Autodesk Inventor part; units mm, degrees
ref_plane "Flange Pattern Plane" through (31.75, 7.5406, -4.5466) normal (0, 1, 0) x (1, 0, 0)
ref_plane "YZ Plane" through (0, 0, 0) normal (1, 0, 0) x (0, 1, 0)
ref_plane "XZ Plane" through (0, 0, 0) normal (0, 1, 0) x (-1, 0, 0)
sketch "Sketch1" plane through (0, 0, 0) normal (0, 1, 0) x (-1, 0, 0)
  line L0 (-31.75, 0) -> (31.75, 0)
  line L1 (31.75, 0) -> (31.75, -12.7)
  line L2 (31.75, -12.7) -> (-31.75, -12.7)
  line L3 (-31.75, -12.7) -> (-31.75, 0)
  line L4 (31.75, 0) -> (-31.75, -12.7) construction
  point P0 (0, 0)
  point P1 (0, 0)
  dimension "d0" = 63.5
  dimension "d1" = 12.7
extrude "Plate1" add sketch "Sketch1" along normal blind 1.1906
sketch "Sketch2" plane through (30.5594, 0, -12.7) normal (1, 0, 0) x (0, 1, 0)
  line L0 (0, 12.7) -> (0, 0)
  line L1 (0, 0) -> (13.8906, 0)
  line L2 (13.8906, 0) -> (13.8906, 12.7)
  line L3 (13.8906, 12.7) -> (0, 12.7)
edge flange "Flanges" height 12.7 angle 90 thickness 1.1906 bend radius 0.7937 thickness toward (1, 0, 0) relief tear relief width 1.1906 relief depth 0.5953 corner gap 1.1906 corner form 0 edges at (31.75, 1.1906, -6.35) (-31.75, 1.1906, -6.35) wall of the first edge with corners at (30.5594, 0, 0) (30.5594, 0, -12.7) (30.5594, 13.8906, -12.7) (30.5594, 13.8906, 0)
bend "Bend1"
corner "Corner1"
sketch "Sketch3" plane through (31.75, 1.9844, -12.7) normal (1, 0, 0) x (0, 0, -1)
  line L0 (-8.1534, 7.8677) -> (-4.5466, 7.8677)
  line L1 (-4.0386, 7.3597) -> (-4.0386, 3.7529)
  line L2 (-4.5466, 3.2449) -> (-8.1534, 3.2449)
  line L3 (-8.6614, 3.7529) -> (-8.6614, 7.3597)
  arc A0 (-8.1534, 7.8677) -> (-8.6614, 7.3597) centre (-8.1534, 7.3597) ccw
  arc A1 (-4.0386, 7.3597) -> (-4.5466, 7.8677) centre (-4.5466, 7.3597) ccw
  arc A2 (-4.5466, 3.2449) -> (-4.0386, 3.7529) centre (-4.5466, 3.7529) ccw
  arc A3 (-8.6614, 3.7529) -> (-8.1534, 3.2449) centre (-8.1534, 3.7529) ccw
  line L4 (-12.7, 0) -> (-12.7, 11.9063) construction
  line L5 (-12.7, 11.9063) -> (0, 11.9063) construction
  line L6 (-8.1534, 7.3597) -> (-4.5466, 3.7529) construction
  point P0 (-12.7, -1.9844)
  point P1 (-4.0386, 3.2449)
  point P2 (-8.6614, 3.2449)
  point P3 (-6.35, 5.5563)
  dimension "d16" = 4.6228
  dimension "d17" = 0.508
  dimension "d20" = 6.35
  dimension "d21" = 6.35
extrude "Flange Stamp" cut sketch "Sketch3" against normal blind 1.1906
sketch "Sketch7" plane through (31.75, 1.9844, 0) normal (1, 0, 0) x (0, 0, -1)
  arc A0 (4.5466, 7.8677) -> (4.0386, 7.3597) centre (4.5466, 7.3597) ccw construction
  arc A1 (8.1534, 3.2449) -> (8.6614, 3.7529) centre (8.1534, 3.7529) ccw construction
  circle A2 centre (6.35, 5.5563) radius 2.1844
  line L0 (4.5466, 7.3597) -> (8.1534, 3.7529) construction
  point P0 (0, -1.9844)
  dimension "d46" = 4.3688
surface extrude "Flange Circle" sketch "Sketch7" against normal up to surface (1.1906 mm away) shown yes curves A2
ref_plane "Flange Pattern Plane" through (31.75, 7.5406, -4.5466) normal (0, 1, 0) x (1, 0, 0)
feature "Flange Pattern" [suppressed]
sketch "Sketch8" plane through (0, 0, 0) normal (0, -1, 0) x (1, 0, 0)
  line L0 (29.7656, 0) -> (-29.7656, 0) construction
  line L1 (27.2034, -4.0386) -> (23.5966, -4.0386)
  line L2 (23.0886, -4.5466) -> (23.0886, -8.1534)
  line L3 (23.5966, -8.6614) -> (27.2034, -8.6614)
  line L4 (27.7114, -8.1534) -> (27.7114, -4.5466)
  arc A0 (27.7114, -4.5466) -> (27.2034, -4.0386) centre (27.2034, -4.5466) ccw
  arc A1 (27.2034, -8.6614) -> (27.7114, -8.1534) centre (27.2034, -8.1534) ccw
  arc A2 (23.0886, -8.1534) -> (23.5966, -8.6614) centre (23.5966, -8.1534) ccw
  arc A3 (23.5966, -4.0386) -> (23.0886, -4.5466) centre (23.5966, -4.5466) ccw
  line L5 (27.2034, -4.5466) -> (23.5966, -8.1534) construction
  line L6 (31.75, 0) -> (31.75, -12.7) construction
  point P0 (0, 0)
  point P1 (23.0886, -8.6614)
  point P2 (27.7114, -8.6614)
  point P3 (25.4, -6.35)
  dimension "d49" = 4.6228
  dimension "d50" = 0.508
  dimension "d51" = 6.35
  dimension "d52" = 6.35
extrude "Body Stamp" cut sketch "Sketch8" against normal blind 1.1906
sketch "Sketch9" plane through (0, 0, 0) normal (0, -1, 0) x (1, 0, 0)
  arc A0 (27.7114, -4.5466) -> (27.2034, -4.0386) centre (27.2034, -4.5466) ccw construction
  arc A1 (23.0886, -8.1534) -> (23.5966, -8.6614) centre (23.5966, -8.1534) ccw construction
  line L0 (27.2034, -4.5466) -> (23.5966, -8.1534) construction
  circle A2 centre (25.4, -6.35) radius 2.1844
  point P0 (0, 0)
  dimension "d55" = 4.3688
surface extrude "Body Circle" sketch "Sketch9" against normal up to surface (1.1906 mm away) shown yes curves A2
feature "Body Pattern" [suppressed]
sketch "Arc Length" plane through (30.5594, 1.9844, 0) normal (0, 0, 1) x (1, 0, 0)
  line L0 (0, 0) -> (1.1906, 0) construction
  arc A0 (-0.7938, -0.7938) -> (0, 0) centre (-0.7938, 0) ccw construction
  line L1 (-0.7938, -1.9844) -> (-0.7938, -0.7938) construction
  arc A1 (-0.7938, -1.9844) -> (1.1906, 0) centre (-0.7938, 0) ccw construction
  point P0 (-30.5594, -1.9844)
  dimension "d85" = 3.117
  dimension "d92" = 1.2468
sketch "Sketch13" plane through (31.75, 13.8906, 0) normal (1, 0, 0) x (0, 0, -1)
  line L0 (0, 0) -> (12.7, 0) construction
  line L1 (62.4078, 0) -> (63.4238, -1.016)
  line L2 (63.4238, -1.016) -> (64.4398, 0)
  line L3 (62.4078, 0) -> (64.4398, 0)
  line L4 (12.7, -11.9063) -> (0, -11.9063) construction
  line L5 (63.4238, -10.8903) -> (61.3168, -12.9972)
  line L6 (61.3168, -12.9972) -> (63.4238, -15.1042)
  line L7 (63.4238, -15.1042) -> (65.5308, -12.9972)
  line L8 (65.5308, -12.9972) -> (63.4238, -10.8903)
  line L9 (63.4238, -10.8903) -> (63.4238, -15.1042) construction
  line L10 (63.4238, -1.016) -> (63.4238, -10.8903) construction
  line L11 (0, -11.9063) -> (12.7, -11.9063) construction
  point P0 (0, -13.8906)
  dimension "d86" = 4.2139
  dimension "d88" = 1.016
  dimension "d91" = 1.016
  dimension "d102" = 63.4238
feature "Notch" [suppressed]
mirror "Notch Mirror" [suppressed]
pattern_linear "Notch Pattern" [suppressed]
chamfer "End Chamfer" distance 1.016 angle 45 4 edges at (-31.1547, 13.8906, -12.7) (31.1547, 13.8906, -12.7) (-31.1547, 13.8906, 0) (31.1547, 13.8906, 0)
sketch "Sketch14" plane through (-31.75, 1.9844, 431.8) normal (1, 0, 0) x (0, 0, -1)
  line L0 (431.8, 11.9063) -> (444.5, 11.9063) construction
  line L1 (431.8, 0) -> (431.8, 11.9063) construction
  line L2 (431.8, -1.9844) -> (444.5, -1.9844) construction
  line L3 (431.8, 11.9063) -> (444.5, 11.9063)
  line L4 (444.5, 11.9063) -> (444.5, -1.9844)
  line L5 (444.5, -1.9844) -> (431.8, -1.9844)
  line L6 (431.8, -1.9844) -> (431.8, 11.9063)
  point P0 (382.0521, -1.9844)
extrude "Half Cut" cut sketch "Sketch14" along normal blind 50.8
sketch "Flange Pattern Sketch" plane through (31.75, 7.5406, -4.5466) normal (0, 1, 0) x (1, 0, 0)
  line L0 (0, 3.6068) -> (0, 0) construction
  line L1 (-76.2822, -4.5466) -> (13.1932, -4.5466) construction
  line L2 (0, 0) -> (-1.1906, 0) construction
  point P0 (-31.75, -4.5466)
  point P1 (0, 1.8034)
  point P2 (0, 14.5034)
  point P3 (0, 27.2034)
  point P4 (0, 39.9034)
  point P5 (0, 52.6034)
  point P6 (0, 65.3034)
  point P7 (0, 78.0034)
  point P8 (0, 90.7034)
  point P9 (0, 103.4034)
  point P10 (0, 116.1034)
  point P11 (0, 128.8034)
  point P12 (0, 141.5034)
  point P13 (0, 154.2034)
  point P14 (0, 166.9034)
  point P15 (0, 179.6034)
  point P16 (0, 192.3034)
  point P17 (0, 205.0034)
  point P18 (0, 217.7034)
  point P19 (0, 230.4034)
  point P20 (0, 243.1034)
  point P21 (0, 255.8034)
  point P22 (0, 268.5034)
  point P23 (0, 281.2034)
  point P24 (0, 293.9034)
  point P25 (0, 306.6034)
  point P26 (0, 319.3034)
  point P27 (0, 332.0034)
  point P28 (0, 344.7034)
  point P29 (0, 357.4034)
  point P30 (0, 370.1034)
  point P31 (0, 382.8034)
  point P32 (0, 395.5034)
  point P33 (0, 408.2034)
  point P34 (0, 420.9034)
  point P35 (0, 433.6034)
  dimension "d131" = 12.7
  dimension "d134" = 12.7
sketch "Body Pattern Sketch" plane through (0, 0, 0) normal (0, -1, 0) x (1, 0, 0)
  line L0 (29.7656, 0) -> (-29.7656, 0) construction
  line L1 (31.75, 0) -> (31.75, -12.7) construction
  circle A0 centre (25.4, -6.35) radius 2.1844 construction
  point P0 (0, 0)
  point P1 (25.4, -19.05)
  point P2 (25.4, -31.75)
  point P3 (25.4, -44.45)
  point P4 (25.4, -57.15)
  point P5 (25.4, -69.85)
  point P6 (25.4, -82.55)
  point P7 (25.4, -95.25)
  point P8 (25.4, -107.95)
  point P9 (25.4, -120.65)
  point P10 (25.4, -133.35)
  point P11 (25.4, -146.05)
  point P12 (25.4, -158.75)
  point P13 (25.4, -171.45)
  point P14 (25.4, -184.15)
  point P15 (25.4, -196.85)
  point P16 (25.4, -209.55)
  point P17 (25.4, -222.25)
  point P18 (25.4, -234.95)
  point P19 (25.4, -247.65)
  point P20 (25.4, -260.35)
  point P21 (25.4, -273.05)
  point P22 (25.4, -285.75)
  point P23 (25.4, -298.45)
  point P24 (25.4, -311.15)
  point P25 (25.4, -323.85)
  point P26 (25.4, -336.55)
  point P27 (25.4, -349.25)
  point P28 (25.4, -361.95)
  point P29 (25.4, -374.65)
  point P30 (25.4, -387.35)
  point P31 (25.4, -400.05)
  point P32 (25.4, -412.75)
  point P33 (25.4, -425.45)
  point P34 (25.4, -438.15)
  dimension "d62" = 12.7
  dimension "d65" = 12.7
  dimension "d139" = 12.7
equation "\"d1\" = 1.27 * Length"
equation "\"d18\" = Thickness"
equation "\"d53\" = Thickness"
equation "\"d89\" = Thickness"
equation "\"d2\" = Thickness"
equation "\"d3\" = BendReliefWidth"
equation "\"d4\" = BendReliefDepth"
equation "\"d5\" = MinimumRemnant"
equation "\"d6\" = TransitionRadius"
equation "\"d10\" = CornerReliefSize"
equation "\"d11\" = GapSize"
equation "\"d12\" = JacobiRadiusSize"
equation "\"BendRadius\" = Thickness"
equation "\"BendReliefWidth\" = Thickness"
equation "\"BendReliefDepth\" = 0.5 * Thickness"
equation "\"CornerReliefSize\" = 4 * Thickness"
equation "\"MinimumRemnant\" = 2 * Thickness"
equation "\"TransitionRadius\" = BendRadius"
equation "\"JacobiRadiusSize\" = BendRadius"
equation "\"GapSize\" = Thickness"
properties part number "Alu C 1x3x1x35"
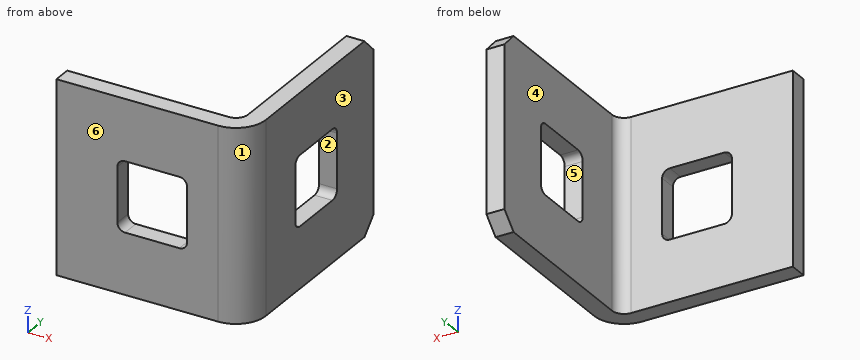
Design review of the part built by this model. Coordinates are the model's own, in mm. Face numbers are marked on the shaded views. A direction names the side the tool comes from. Give positions to 0.01 mm unless a question says otherwise; leave off trailing zeros. Write each loop counter-clockwise with the first axis right and the second up, starting at its lowest first coordinate (ties: lowest second). Pieces come first, ordered by that corner, then holes. Notation, with made-up numbers: M 73,37.5 L 103,37.5 A19 ccw 103,66.5 Z; hole C -4.75,46 d2. An arc over 180 degrees is marked long. Return JSON: item names as keys, results as strings. Group by question number.
Item 1: Take a section at C-C (y = 6). Give the boundary of the cut face in (x, z).
Item 2: Wall thickness on line 1 along Y through (x, z) = (26.25, -4); line 2 along X through (y, z) = (9, -1.25); line 3 along Y through (x, z) = (30.25, -3.5): over which ranges is each line inside the solid? List them lowest first.
Item 3: Take a section at D-D (z = -10.5). Give the boundary of the cut face in (x, y), plus the area to 3 significant figures.
Item 4: Tool access review of the marked faces 4, 5 and 6: name each direction out of +Z, -Z, +X, -X, +Y, -Y from which nothing blocks a thin tool from reaching the whole face with its end or side.
Item 5: Take a section at B-B (z = -6.5). Give the boundary of the cut face in (x, y), plus the area to 3 significant figures.
Item 6: Clearance check with flat-ended pins moving along their axes: pin 1 Ø1 at (x, y) = (26, 3) entering from +Z; pin 2 Ø3 at (x, y) = (30.5, 4.5) entering from -Z; pin 3 Ø1.5 at (y, z) = (3.5, -9) entering from -X; pin 4 Ø5 at (x, z) = (25.5, -2) entering from +Y. State where each tip first meets the part, or that it passes through.
Item 7: Take a section at A-A (x = 24). Give the boundary of the cut face in (y, z), plus the area to 3 significant figures.
Item 8: The part is to be moulded in two halves that separate along Y. For the marked faces 1, 2 and 3, say which applies: pulls with the +Y half, pulls with the -Y half, needs draft (parallel to the pull), parting line crosses it, or undercut.
Return value:
{
 "1": {"outline": "M 30.56,-12.7 L 31.75,-12.7 L 31.75,-8.66 L 30.56,-8.66 Z; M 30.56,-4.04 L 31.75,-4.04 L 31.75,0 L 30.56,0 Z"},
 "2": {"line 1": "y = 0 to 1.19", "line 2": "x = 30.56 to 31.75", "line 3": "y = 0.06 to 1.36"},
 "3": {"outline": "M 19.05,0 L 29.77,0 A1.98 ccw 31.75,1.98 L 31.75,13.89 L 30.56,13.89 L 30.56,1.98 A0.79 cw 29.77,1.19 L 19.05,1.19 Z", "area": "29.5 mm2"},
 "4": {"face 4": "+Z, -Z, -X, +Y", "face 5": "+X, -X", "face 6": "+Z, -Z, +X, -X, -Y"},
 "5": {"outline": "M 19.05,0 L 23.09,0 L 23.09,1.19 L 19.05,1.19 Z; M 27.71,0 L 29.77,0 A1.98 ccw 31.75,1.98 L 31.75,5.23 L 30.56,5.23 L 30.56,1.98 A0.79 cw 29.77,1.19 L 27.71,1.19 Z; M 30.56,9.85 L 31.75,9.85 L 31.75,13.89 L 30.56,13.89 Z", "area": "18.5 mm2"},
 "6": {"pin 1": "passes through", "pin 2": "stops at z = -12.7", "pin 3": "stops at x = 30.56", "pin 4": "stops at y = 1.19"},
 "7": {"outline": "M 0,-12.7 L 1.19,-12.7 L 1.19,-8.66 L 0,-8.66 Z; M 0,-4.04 L 1.19,-4.04 L 1.19,0 L 0,0 Z", "area": "9.62 mm2"},
 "8": {"face 1": "pulls with the -Y half", "face 2": "undercut", "face 3": "needs draft"}
}
